Design review of the part built by this model. Coordinates are the model's own, in mm. A direction names the side the tool comes from. Coordinates: 2 decimals unless noted, no trailing zeros. Loops run counter-clockwise (first coordinate to the right, second up) from the corner with the lowest first, then second, coordinate; pieces in that order, holes last. Notation, with made-up numbers: (78.5, 28) -> (132.5, 28) arc R30 cw to (132.5, 63) -> close; hole circle Ø11 at (11, 62.25). An arc over 180 degrees is marked (long way). Use a Markdown table: item, result. Add a question column.
Q1. Take a section at B-B on y = 4.5. Write out the cut boundary in (x, z), plus the area to 3 significant figures.
Q2. For probe 1 along Y at (x, z) = (36.5, 0.6); probe 2 along X at (y, z) = (3, 6); probe 3 along Z at (x, y) = (44, 1.5), list the stretches that pass through material, from the lowest coordinate up.
Q3. Take a section at A-A on z = 2.75. Write out the cut boundary in (x, y), plus the area to 3 significant figures.
Q4. Clearance check with flat-ended pins moving along their axes: pin 1 Ø1 at (y, z) = (4.5, 5.5) entering from -X; pin 2 Ø2 at (x, y) = (34, 4) entering from +Z; pin 3 Ø1.1 at (y, z) = (4.5, 4.5) entering from +X. State where each tip first meets the part, or that it passes through.
Q5. Draft analysis for pull direction X (two halves, no side actions). For faces 4 (the face through (0, 1, 5)), 5 (the face through (26, 8, 6)), 6 (the face through (18, 4, 1)), state which applies: pulls with the +X half, pulls with the -X half, needs draft (parallel to the pull), parting line crosses it, or undercut.
Q6. For faces 1 (the face through (46, 5, 4.2)), 2 (the face through (44.5, 1, 3)), 3 (the face through (43, 4, 6)), list the 3-axis set-ups (+Z, -Z, +X, -X, +Y, -Y) from which the entire face can be reached by the end or side of a thin tool; tool diameter is ignored.
Q7. Take a section at D-D on y = 2.5. Write out the cut boundary in (x, z).
Q8. Take a section at C-C on x = 8. Write out the cut boundary in (y, z).
from build123d import *

# Parameters (mm, degrees)
SKETCH_1_W             = 52
SKETCH_1_H             = 9
EXTRUDE_1_DEPTH        = 2
SKETCH_1_5_W           = 1
SKETCH_1_5_H           = 7
SKETCH_1_5_W_2         = 1.5
SKETCH_1_5_H_2         = 1
CUT_EXTRUDE_2_DEPTH    = 53.810983706
EXTRUDE_START          = 2
SKETCH_1_6_W           = 6
SKETCH_1_6_H           = 2.8
EXTRUDE_2_DEPTH        = 6
PATTERN_LINEAR_1_COUNT = 3
PATTERN_LINEAR_1_PITCH = 20
SKETCH_1_7_W           = 5
SKETCH_1_7_H           = 2
EXTRUDE_3_DEPTH        = 5
SKETCH_2_R             = 1.5
CUT_EXTRUDE_3_DEPTH    = 54.075418039


with BuildPart() as part:
    # 草图1 → 凸台-拉伸1 (new body)
    with BuildSketch(Plane(origin=(0, 0, 0), x_dir=(1, 0, 0), z_dir=(0, 1, 0))):
        with Locations((26, -4.5)):
            Rectangle(SKETCH_1_W, SKETCH_1_H)
    extrude(amount=EXTRUDE_1_DEPTH)

    # 草图1<5> → 切除-拉伸2 (cut, through all)
    with BuildSketch(Plane(origin=(0, 0, 0), x_dir=(1, 0, 0), z_dir=(0, 1, 0))):
        with Locations((9.5, -3.5)):
            Rectangle(SKETCH_1_5_W, SKETCH_1_5_H)
        with Locations((2.5, -3.5)):
            Rectangle(SKETCH_1_5_W, SKETCH_1_5_H)
        with Locations((3.75, -2.7)):
            Rectangle(SKETCH_1_5_W_2, SKETCH_1_5_H_2)
        with Locations((8.25, -2.7)):
            Rectangle(SKETCH_1_5_W_2, SKETCH_1_5_H_2)
    cut_extrude_2 = extrude(amount=CUT_EXTRUDE_2_DEPTH, mode=Mode.SUBTRACT)

    # 草图1<6> → 凸台-拉伸2 (add)
    with BuildSketch(Plane(origin=(0, 0, 0), x_dir=(1, 0, 0), z_dir=(0, 1, 0)).offset(EXTRUDE_START)):
        with Locations((6, -5.6)):
            Rectangle(SKETCH_1_6_W, SKETCH_1_6_H)
    extrude_2 = extrude(amount=EXTRUDE_2_DEPTH)

    # 阵列(线性)1: 切除-拉伸2, 凸台-拉伸2 ×3
    with Locations(*[(i * PATTERN_LINEAR_1_PITCH, 0, 0) for i in range(1, PATTERN_LINEAR_1_COUNT)]):
        add(cut_extrude_2, mode=Mode.SUBTRACT)
        add(extrude_2)

    # 草图1<7> → 凸台-拉伸3 (add)
    with BuildSketch(Plane(origin=(0, 0, 0), x_dir=(1, 0, 0), z_dir=(0, 1, 0)).offset(EXTRUDE_START)):
        with Locations((15.5, -1)):
            Rectangle(SKETCH_1_7_W, SKETCH_1_7_H)
        with Locations((36.5, -1)):
            Rectangle(SKETCH_1_7_W, SKETCH_1_7_H)
    extrude(amount=EXTRUDE_3_DEPTH)

    # 草图2 → 切除-拉伸3 (cut, through all)
    with BuildSketch(Plane.XY.offset(2)):
        with Locations((36.5, 4.5)):
            Circle(SKETCH_2_R)
        with Locations((15.5, 4.5)):
            Circle(SKETCH_2_R)
    extrude(amount=-CUT_EXTRUDE_3_DEPTH, mode=Mode.SUBTRACT)


solid = part.part
Answer list:
| question | item | result |
|---|---|---|
| 1 | outline | (3, 4.2) -> (9, 4.2) -> (9, 7) -> (3, 7) -> close; (13, 0) -> (14, 0) -> (14, 2) -> (13, 2) -> close; (17, 0) -> (18, 0) -> (18, 2) -> (17, 2) -> close; (23, 4.2) -> (29, 4.2) -> (29, 7) -> (23, 7) -> close; (34, 0) -> (35, 0) -> (35, 2) -> (34, 2) -> close; (38, 0) -> (39, 0) -> (39, 2) -> (38, 2) -> close; (43, 4.2) -> (49, 4.2) -> (49, 7) -> (43, 7) -> close |
| 1 | area | 58.4 mm² |
| 2 | probe 1 | 0 to 3, 6 to 7 |
| 2 | probe 2 | 3 to 9, 23 to 29, 43 to 49 |
| 2 | probe 3 | 0 to 2.2, 3.2 to 9 |
| 3 | outline | (0, 0) -> (2, 0) -> (2, 2) -> (0, 2) -> close; (4.5, 0) -> (7.5, 0) -> (7.5, 2) -> (4.5, 2) -> close; (10, 0) -> (22, 0) -> (22, 2) -> (10, 2) -> close; (24.5, 0) -> (27.5, 0) -> (27.5, 2) -> (24.5, 2) -> close; (30, 0) -> (42, 0) -> (42, 2) -> (30, 2) -> close; (44.5, 0) -> (47.5, 0) -> (47.5, 2) -> (44.5, 2) -> close; (50, 0) -> (52, 0) -> (52, 2) -> (50, 2) -> close |
| 3 | area | 74.0 mm² |
| 4 | pin 1 | x = 3 |
| 4 | pin 2 | z = 2 |
| 4 | pin 3 | x = 49 |
| 5 | face 4 | pulls with the -X half |
| 5 | face 5 | needs draft |
| 5 | face 6 | undercut |
| 6 | face 1 | -Z, +X, -X, +Y |
| 6 | face 2 | +Y, -Y |
| 6 | face 3 | -Z, +Y, -Y |
| 7 | outline | (3, 4.2) -> (9, 4.2) -> (9, 7) -> (3, 7) -> close; (13, 0) -> (18, 0) -> (18, 2) -> (13, 2) -> close; (23, 4.2) -> (29, 4.2) -> (29, 7) -> (23, 7) -> close; (34, 0) -> (39, 0) -> (39, 2) -> (34, 2) -> close; (43, 4.2) -> (49, 4.2) -> (49, 7) -> (43, 7) -> close |
| 8 | outline | (0, 0) -> (2, 0) -> (2, 2.2) -> (0, 2.2) -> close; (0, 3.2) -> (2, 3.2) -> (2, 4.2) -> (8, 4.2) -> (8, 7) -> (2, 7) -> (2, 9) -> (0, 9) -> close |
